Source: CAD feature listing. Evaluate the final solid. Frame: model axes, mm. A direction names the side the tool comes from. Coordinates: 2 decimals unless noted, no trailing zeros. Order: outer loops, then holes, each group sorted by start corner. A loop starts at its lowest first (then second) coordinate and runs counter-clockwise, first axis right, second up.
```python
from build123d import *

# Parameters (mm, degrees)
F1_DEPTH = 12.7
F2_R     = 1.905
F3_DEPTH = 3.81
F4_R     = 1.905
F5_DEPTH = 3.81


with BuildPart() as f1:
    # F0 (on Top) → F1 (new body)
    with BuildSketch(Plane.XY):
        Polygon((18.936607, 16.403033), (-26.783393, 16.403033), (-26.783393, 31.643033), (-30.593393, 31.643033), (-30.593393, 16.403033), (-30.593393, 12.593033), (15.126607, 12.593033), (15.126607, -35.539288), (8.47132, -35.539288), (8.47132, -39.349288), (8.47132, -50.648663), (12.28132, -50.648663), (12.28132, -39.349288), (18.979067, -39.349288), (18.936607, -35.848397), (18.936607, 12.593033), align=None)
    extrude(amount=F1_DEPTH)

    # F2 (on face) → F3 (cut, through all)
    with BuildSketch(Plane.YZ.offset(12.28132)):
        with Locations((-44.998975, 6.59027)):
            Circle(F2_R)
    extrude(amount=-F3_DEPTH, mode=Mode.SUBTRACT)

    # F4 (on face) → F5 (cut, through all)
    with BuildSketch(Plane(origin=(-30.593393, 0, 0), x_dir=(0, -1, 0), z_dir=(-1, 0, 0))):
        with Locations((-25.961572, 6.35)):
            Circle(F4_R)
    extrude(amount=-F5_DEPTH, mode=Mode.SUBTRACT)


solid = f1.part
```
Q1. Material intervals for line 1 along Y through (x, z) = (14.5, 1.25); line 2 along Y through (x, z) = (7, 6.5); line 3 along Y through (x, z) = (11, 11), sorted ascending.
Solutions:
line 1: y = -39.35 to -35.54, 12.59 to 16.4
line 2: y = 12.59 to 16.4
line 3: y = -50.65 to -35.54, 12.59 to 16.4
Q2. Pin query (flat end, axial travel): P1, Ø6, axis at x = 2.5, z = 6, coming from the +Y side; P2, Ø6.5, axis at y = -6.5, z = 6.5, coming from the -X side; P3, Ø6.5, axis at y = -17, z = 9, coming from the +X side; P4, Ø3.5, axis at y = -45, z = 6.59, coming from the +X side. Return the tip coordinate at first contact, or that it passes through.
Solutions:
P1: stops at y = 16.4
P2: stops at x = 15.13
P3: stops at x = 18.94
P4: passes through
Q3. Section query B-B on x = 9.5. Output: boundary loops of the cut face in (y, z) (3 decimals).
Solutions:
outline: (-50.649, 0) - (-35.539, 0) - (-35.539, 12.7) - (-50.649, 12.7) - close; (12.593, 0) - (16.403, 0) - (16.403, 12.7) - (12.593, 12.7) - close; hole circle Ø3.81 at (-44.999, 6.59)
Q4. Section query D-D on x = -23. Output: boundary loops of the cut face in (y, z).
Solutions:
outline: (12.59, 0) - (16.4, 0) - (16.4, 12.7) - (12.59, 12.7) - close
Q5. Section query C-C on z = 10.75. Output: boundary loops of the cut face in (x, y), plus the area to 3 significant figures.
Solutions:
outline: (-30.59, 12.59) - (15.13, 12.59) - (15.13, -35.54) - (8.47, -35.54) - (8.47, -50.65) - (12.28, -50.65) - (12.28, -39.35) - (18.98, -39.35) - (18.94, -35.85) - (18.94, 16.4) - (-26.78, 16.4) - (-26.78, 31.64) - (-30.59, 31.64) - close
area: 513 mm2
Q6. Pull-direction query (Y, two-part tool) for faces 5 (the flat face through (16, -3, 12.7)), 6 (the flat face through (16, -39.349, 6)), 7 (the cylindrical face through (10.4, -46.9, 6.7)); classes: pulls with the +Y half, pulls with the -Y half, needs draft (parallel to the pull), parting line crosses it, or undercut.
Solutions:
face 5: needs draft
face 6: pulls with the -Y half
face 7: undercut
Q7. Section query A-A on y = 25. Output: boundary loops of the cut face in (x, z).
Solutions:
outline: (-30.59, 0) - (-26.78, 0) - (-26.78, 4.71) - (-30.59, 4.71) - close; (-30.59, 7.99) - (-26.78, 7.99) - (-26.78, 12.7) - (-30.59, 12.7) - close
Q8. Set-up query: faces 1 (the flat face through (-26.783, 23.9, 6.3)), 2 (the flat face through (15.127, -11, 6)), 3 (the flat face through (8.471, -43, 6)), 4 (the flat face through (12.281, -43.8, 4.8)). Return all of +Z, -Z, +X, -X, +Y, -Y with unobstructed straight access to the full face (end or side cutting, diameter ignored); none if empty.
Solutions:
face 1: +Z, -Z, +X, +Y
face 2: +Z, -Z, -X
face 3: +Z, -Z, -X, -Y
face 4: +Z, -Z, +X, -Y
